Design review of the part built by this model. Coordinates are the model's own, in mm. Coordinates: 2 decimals unless noted, no trailing zeros. Loops run counter-clockwise (first coordinate to the right, second up) from the corner with the lowest first, then second, coordinate; pieces in that order, holes last. Notation, with made-up numbers: (-2.75, 1) -> (37.25, 1) arc R20 cw to (37.25, 36) -> close; hole circle Ø1 at (83.25, 14). An arc over 180 degrees is marked (long way). Use a Markdown table: item, result. Add a question column.
Q1. Clearance check with a flat-ended pin moving along its axis: pin 1 Ø6.5 at (y, z) = (-41, 41) entering from +X. State where the tip first meets the part, or that it passes through.
Q2. Take a section at A-A on x = 1.7. Write out the cut boundary in (y, z).
Q3. For probe 1 along Y at (x, z) = (0.85, 41); probe 2 along Y at (x, z) = (1.15, 20), list the stretches that pass through material, from the lowest coordinate up.
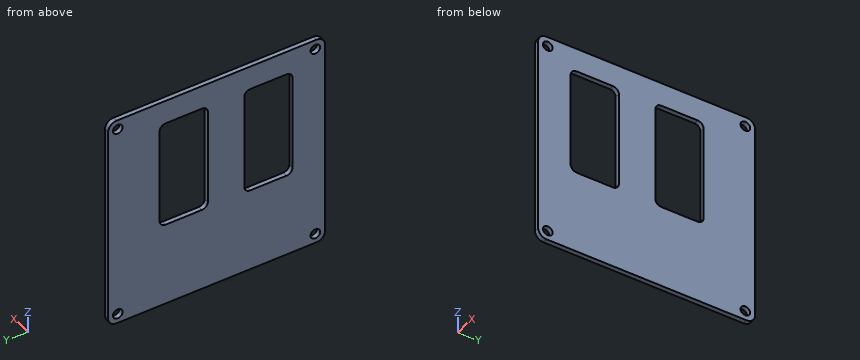
Autodesk Inventor part; units mm, degrees
ref_plane "YZ Plane" through (0, 0, 0) normal (1, 0, 0) x (0, 1, 0)
ref_plane "XZ Plane" through (0, 0, 0) normal (0, 1, 0) x (-1, 0, 0)
ref_plane "XY Plane" through (0, 0, 0) normal (0, 0, 1) x (1, 0, 0)
sketch "Sketch1" plane through (0, 0, 0) normal (1, 0, 0) x (0, 1, 0)
  line L0 (45, 45) -> (-45, 45)
  line L1 (-45, 45) -> (-45, -45)
  line L2 (-45, -45) -> (45, -45)
  line L3 (45, -45) -> (45, 45)
  line L4 (45, 45) -> (-45, -45) construction
  line L5 (-45, 45) -> (45, -45) construction
  point P0 (0, 0)
  dimension "d0" = 90
  dimension "d1" = 90
extrude "Extrusion1" add sketch "Sketch1" along normal blind 2
sketch "Sketch2" plane through (2, 0, 0) normal (1, 0, 0) x (0, 0, -1)
  line L0 (45, 45) -> (-45, 45)
  line L1 (-45, 45) -> (-41, 45)
  line L2 (-41, 45) -> (-41, 41)
  circle A0 centre (-41, 41) radius 2
  line L3 (45, -45) -> (45, 45)
  line L4 (45, 45) -> (41, 45)
  line L5 (41, 45) -> (41, 41)
  circle A1 centre (41, 41) radius 2
  line L6 (-45, 45) -> (-45, -45)
  line L7 (-45, -45) -> (-41, -45)
  line L8 (-45, -45) -> (45, -45)
  line L9 (-41, -45) -> (-41, -41)
  circle A2 centre (-41, -41) radius 2
  line L10 (45, -45) -> (41, -45)
  line L11 (41, -45) -> (41, -41)
  circle A3 centre (41, -41) radius 2
  point P0 (0, 0)
  dimension "d4" = 4
  dimension "d5" = 4
  dimension "d6" = 4
  dimension "d7" = 4
  dimension "d8" = 4
  dimension "d9" = 4
  dimension "d10" = 4
  dimension "d11" = 4
  dimension "d12" = 4
  dimension "d13" = 4
  dimension "d14" = 4
  dimension "d15" = 4
extrude "Extrusion2" cut sketch "Sketch2" against normal up to surface (2 mm away) contours A1 | A0 | A2 | A3
fillet "Fillet1" radius 3.5 4 edges at (1, 45, -45) (1, -45, -45) (1, -45, 45) (1, 45, 45)
sketch "Sketch3" plane through (2, 0, 0) normal (1, 0, 0) x (0, 0, -1)
  line L0 (-41.5, -45) -> (41.5, -45)
  line L1 (0, -45) -> (0, -41.5)
  line L2 (0, -41.5) -> (0, -31.5)
  line L3 (0, -31.5) -> (0, -11.5)
  line L4 (0, -45) -> (0, -6.37)
  line L5 (0, -6.37) -> (0, 3.63)
  line L6 (0, 3.63) -> (0, 23.63)
  line L7 (45, -41.5) -> (45, 41.5)
  line L8 (45, 0) -> (10, 0)
  line L9 (10, 0) -> (10, 3.63)
  line L10 (10, 3.63) -> (-35, 3.63)
  line L11 (-35, 3.63) -> (-35, 23.63)
  line L12 (-35, 23.63) -> (10, 23.63)
  line L13 (10, 23.63) -> (10, 3.63)
  line L14 (10, 0) -> (10, -11.5)
  line L15 (10, -11.5) -> (-35, -11.5)
  line L16 (-35, -11.5) -> (-35, -31.5)
  line L17 (-35, -31.5) -> (10, -31.5)
  line L18 (10, -31.5) -> (10, -11.5)
  point P0 (0, 0)
  dimension "d19" = 3.5
  dimension "d20" = 10
  dimension "d21" = 20
  dimension "d22" = 38.63
  dimension "d23" = 10
  dimension "d24" = 20
  dimension "d25" = 35
  dimension "d26" = 45
  dimension "d27" = 20
  dimension "d28" = 45
  dimension "d29" = 20
extrude "Extrusion3" cut sketch "Sketch3" against normal up to surface (2 mm away) contours L17 L16 L15 L3 | L3 L15 L18 L17 | L10 L11 L12 L6 | L6 L12 L13 L10
fillet "Fillet2" radius 2.5 8 edges at (1, 23.63, -10) (1, -11.5, -10) (1, 23.63, 35) (1, -11.5, 35) (1, 3.63, -10) (1, -31.5, -10) (1, 3.63, 35) (1, -31.5, 35)
properties part number "RightCover" material "ABS Plastic"
Answer list:
| question | item | result |
|---|---|---|
| 1 | pin 1 | x = 2 |
| 2 | outline | (-45, -41.5) arc R3.5 ccw to (-41.5, -45) -> (41.5, -45) arc R3.5 ccw to (45, -41.5) -> (45, 41.5) arc R3.5 ccw to (41.5, 45) -> (-41.5, 45) arc R3.5 ccw to (-45, 41.5) -> close; hole circle Ø4 at (-41, -41); hole circle Ø4 at (-41, 41); hole (-31.5, -7.5) arc R2.5 ccw to (-29, -10) -> (-14, -10) arc R2.5 ccw to (-11.5, -7.5) -> (-11.5, 32.5) arc R2.5 ccw to (-14, 35) -> (-29, 35) arc R2.5 ccw to (-31.5, 32.5) -> close; hole (3.63, -7.5) arc R2.5 ccw to (6.13, -10) -> (21.13, -10) arc R2.5 ccw to (23.63, -7.5) -> (23.63, 32.5) arc R2.5 ccw to (21.13, 35) -> (6.13, 35) arc R2.5 ccw to (3.63, 32.5) -> close; hole circle Ø4 at (41, -41); hole circle Ø4 at (41, 41) |
| 3 | probe 1 | -45 to -43, -39 to 39, 43 to 45 |
| 3 | probe 2 | -45 to -31.5, -11.5 to 3.63, 23.63 to 45 |
